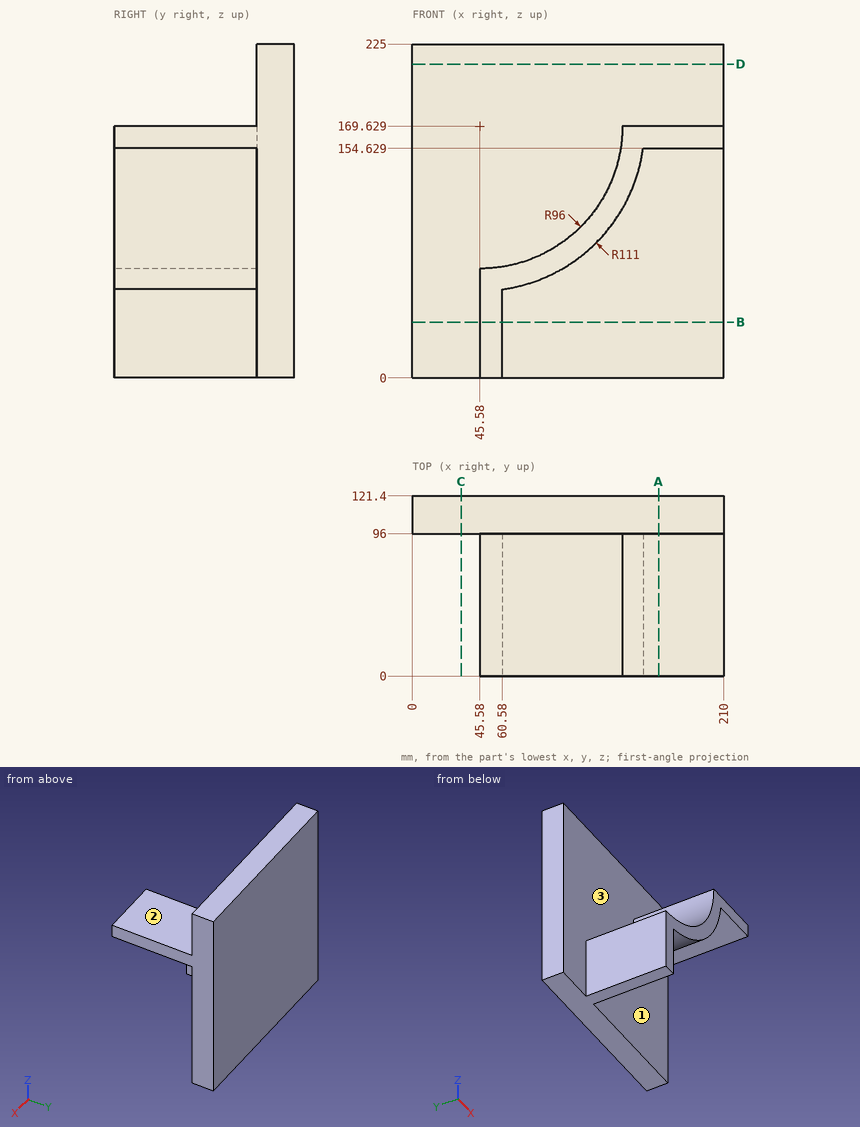
Design review of the part shown in the three views and the two pictorial views. Dimensions are in mm from the part's minimum x, y and z. A direction names the side the tool comes from. Round coordinates to 2 decimals unless told otherwise and drop trailing zeros. Loops run counter-clockwise (first coordinate to the right, second up) from the corner with the lowest first, then second, coordinate; pieces in that order, holes last. Notation, with made-up numbers: (16.25, -22) - (46.25, -22) arc R9 cw to (46.25, -6) - close; hole circle Ø2 at (-23.5, -31). An arc over 180 degrees is marked (long way). Answer as CSV lines item,"result".
(1) Consider section C-C on x = 33. Give the boundary of the cut face in (y, z), then the cut area to 4 significant figures.
Checked values:
outline,"(96, 0) - (121.4, 0) - (121.4, 225) - (96, 225) - close"
area,"5,715 mm2"
(2) Insertion check: P1, Ø2, axis at x = 101.5, z = 47, coming from the -Y side; P2, Ø4, axis at y = 40, z = 65, coming from the +X side; P3, Ø1, axis at y = 40.5, z = 94, coming from the +X side. Each pin has a flat end and moves straight along its axis. Give the tip position at first contact, or say it passes through.
Checked values:
P1,"stops at y = 96"
P2,"stops at x = 87.87"
P3,"stops at x = 127.29"
(3) Consider section B-B on z = 37.5. Give the boundary of the cut face in (x, y), then the cut area to 3 significant figures.
Checked values:
outline,"(0, 96) - (45.58, 96) - (45.58, 0) - (60.58, 0) - (60.58, 96) - (210, 96) - (210, 121.4) - (0, 121.4) - close"
area,"6,770 mm2"
(4) Consider section A-A on x = 166. Give the boundary of the cut face in (y, z), then the cut area to 4 significant figures.
Checked values:
outline,"(0, 154.63) - (96, 154.63) - (96, 0) - (121.4, 0) - (121.4, 225) - (96, 225) - (96, 169.63) - (0, 169.63) - close"
area,"7,155 mm2"
(5) Consider section D-D on z = 211.5. Give the boundary of the cut face in (x, y).
Checked values:
outline,"(0, 96) - (210, 96) - (210, 121.4) - (0, 121.4) - close"
(6) Tool access review of the marked faces 1, 2 and 3: name each direction out of +Z, -Z, +X, -X, +Y, -Y from which nothing blocks a thin tool from reaching the whole face with its end or side.
Checked values:
face 1,"-Z, +X, -Y"
face 2,"+Z, +X, -X, -Y"
face 3,"+Z, -X, -Y"
(7) Wall thickness on line 1 (Y direction, x = 63, z = 95); line 2 (Z direction, x = 171, y = 11.5); line 3 (X direction, y = 92.5, z = 32.5): over which ranges is each line inside the solid? List them lowest first.
Checked values:
line 1,"y = 96 to 121.4"
line 2,"z = 154.63 to 169.63"
line 3,"x = 45.58 to 60.58"
